Geometry: final body of the model. Coordinates: model frame, mm. Face numbers are marked on the shaded views. Coordinates: 2 decimals unless noted, no trailing zeros. Write each loop counter-clockwise with the first axis right and the second up, starting at its lowest first coordinate (ties: lowest second). Pieces come first, ordered by that corner, then holes. Notation, with made-up numbers: (89, 7.25) - (106, 7.25) arc R13 ccw to (106, 25.25) - close; hole circle Ø9 at (36.5, 57). An arc over 180 degrees is marked (long way). Put each result on its own line as item: value.
Autodesk Inventor part; units mm, degrees
ref_plane "2_to_1_XY" through (0, 0, 20.5) normal (0, 0, 1) x (1, 0, 0)
ref_plane "2_to_1_YZ" through (0, 0, 20.5) normal (1, 0, 0) x (0, 1, 0)
ref_plane "2_to_1_ZX" through (0, 0, 20.5) normal (0, 1, 0) x (0, 0, 1)
sketch "Sketch_1" plane through (0, 0, 0) normal (0, 0, 1) x (1, 0, 0)
  arc A0 (3.7947, -2.6) -> (0, -4.6) centre (0, 0) ccw
  line L0 (0, -4.6) -> (18, -4.6)
  line L1 (18, -4.6) -> (18, -2.6)
  line L2 (18, -2.6) -> (3.7947, -2.6)
  circle A1 centre (0, 0) radius 2.5
extrude "Extrusion1" add sketch "Sketch_1" along normal blind 41
sketch "Sketch_2" plane through (0, -4.6, 0) normal (0, 1, 0) x (1, 0, 0)
  line L0 (9.2, -41) -> (9.2, -43)
  line L1 (9.2, -43) -> (20, -43)
  line L2 (20, -43) -> (20, 2)
  line L3 (20, 2) -> (9.2, 2)
  line L4 (9.2, 2) -> (9.2, 0)
  line L5 (9.2, 0) -> (14, 0)
  arc A0 (18, -4) -> (14, 0) centre (14, -4) ccw
  line L6 (18, -4) -> (18, -37)
  arc A1 (14, -41) -> (18, -37) centre (14, -37) ccw
  line L7 (14, -41) -> (9.2, -41)
extrude "Extrusion2" cut sketch "Sketch_2" along normal blind 2
sketch "Sketch_7" plane through (0, 0, 20.5) normal (0, 0, 1) x (1, 0, 0)
  arc A0 (4.6, 0) -> (0, -4.6) centre (0, 0) ccw
  line L0 (0, -4.6) -> (4.6, -4.6)
  line L1 (4.6, -4.6) -> (4.6, 0)
extrude "Extrusion3" cut sketch "Sketch_7" against normal blind 10.25
sketch "Sketch_5" plane through (0, 0, 41) normal (0, 0, 1) x (1, 0, 0)
  arc A0 (4.6, 0) -> (0, -4.6) centre (0, 0) ccw
  line L0 (0, -4.6) -> (4.6, -4.6)
  line L1 (4.6, -4.6) -> (4.6, 0)
extrude "Extrusion4" cut sketch "Sketch_5" against normal blind 10.25
sketch "Sketch_3" plane through (0, -4.6, 0) normal (0, 1, 0) x (1, 0, 0)
  arc A0 (10, -5.25) -> (10, -10.75) centre (10, -8) ccw
  line L0 (10, -10.75) -> (11, -10.75)
  arc A1 (11, -10.75) -> (11, -5.25) centre (11, -8) ccw
  line L1 (11, -5.25) -> (10, -5.25)
extrude "Extrusion5" cut sketch "Sketch_3" along normal blind 2
sketch "Sketch_4" plane through (0, -4.6, 0) normal (0, 1, 0) x (1, 0, 0)
  arc A0 (10, -30.25) -> (10, -35.75) centre (10, -33) ccw
  line L0 (10, -35.75) -> (11, -35.75)
  arc A1 (11, -35.75) -> (11, -30.25) centre (11, -33) ccw
  line L1 (11, -30.25) -> (10, -30.25)
extrude "Extrusion6" cut sketch "Sketch_4" along normal blind 2
ref_plane "2_to_1_XY" through (0, 0, 20.5) normal (0, 0, 1) x (1, 0, 0)
ref_plane "2_to_1_YZ" through (0, 0, 20.5) normal (1, 0, 0) x (0, 1, 0)
ref_plane "2_to_1_ZX" through (0, 0, 20.5) normal (0, 1, 0) x (0, 0, 1)
properties part number "SHPSNA5_2"
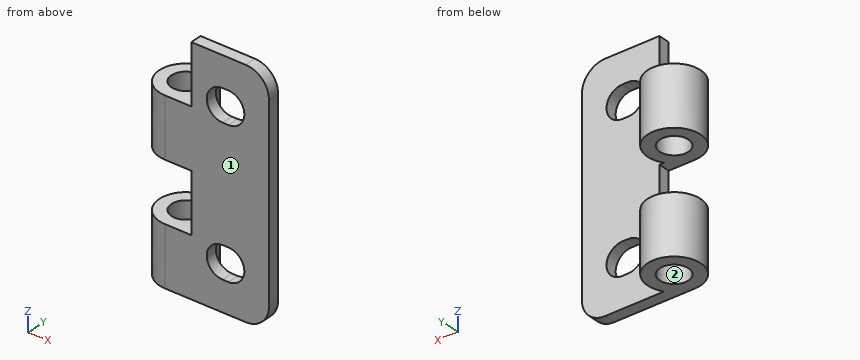
1. Section query A-A (z = 8). Return loops of the section in (x, y).
Answer below:
outline: (0, -4.6) - (7.25, -4.6) - (7.25, -2.6) - (3.79, -2.6) arc R4.6 ccw (long way) to start; (13.75, -4.6) - (18, -4.6) - (18, -2.6) - (13.75, -2.6) - close; hole circle Ø5 at (0, 0)
2. Section query D-D (z = 33). Return loops of the section in (x, y), then the cut area to 3 significant figures.
Answer below:
outline: (4.6, -4.6) - (7.25, -4.6) - (7.25, -2.6) - (4.6, -2.6) - close; (13.75, -4.6) - (18, -4.6) - (18, -2.6) - (13.75, -2.6) - close
area: 13.8 mm²
3. Pin query (flat end, axial travel): pin 1 Ø5 at (x, z) = (3, 31.5) entering from -Y; pin 2 Ø1 at (y, z) = (2, 7) entering from +X; pin 3 Ø1 at (y, z) = (-3.5, 17.5) entering from -X; pin 4 Ø2 at (x, z) = (4.5, 4.5) entering from +Y. Return the tip coordinate at first contact, or that it passes through.
Answer below:
pin 1: stops at y = -4.6
pin 2: stops at x = 4.35
pin 3: stops at x = 4.6
pin 4: stops at y = 2.98
4. Ray query, probe 1 along Y at (x, z) = (0, 27.5); probe 2 along Z at (x, y) = (-3, -2.75). Return the intervals inside material, ascending. Write a range as from..to.
Answer below:
probe 1: y = -4.6..-2.5, 2.5..4.6
probe 2: z = 0..10.25, 20.5..30.75
5. Section query C-C (x = 2). Return loops of the section in (y, z).
Answer below:
outline: (-4.6, 0) - (-1.5, 0) - (-1.5, 10.25) - (-4.6, 10.25) - close; (-4.6, 20.5) - (-1.5, 20.5) - (-1.5, 30.75) - (-4.6, 30.75) - close; (1.5, 0) - (4.14, 0) - (4.14, 10.25) - (1.5, 10.25) - close; (1.5, 20.5) - (4.14, 20.5) - (4.14, 30.75) - (1.5, 30.75) - close
6. Section query B-B (y = 0). Return loops of the section in (x, z).
Answer below:
outline: (-4.6, 0) - (-2.5, 0) - (-2.5, 10.25) - (-4.6, 10.25) - close; (-4.6, 20.5) - (-2.5, 20.5) - (-2.5, 30.75) - (-4.6, 30.75) - close; (2.5, 0) - (4.6, 0) - (4.6, 10.25) - (2.5, 10.25) - close; (2.5, 20.5) - (4.6, 20.5) - (4.6, 30.75) - (2.5, 30.75) - close
7. Mould query, pull axis Y, two halves, no side actions, for the marked faces 1 and 2. Classes: +Y half, -Y half, draft (parallel to the pull), parting line (faces both ways), or undercut.
Answer below:
face 1: -Y half
face 2: undercut
